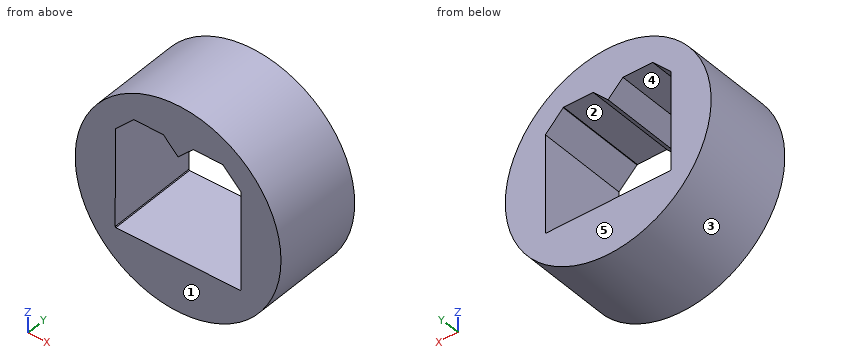
Autodesk Fusion 360 part; units mm, degrees
sketch "Sketch1" plane through (0, 0, 0) normal (0, 1, 0) x (1, 0, 0)
  circle A0 centre (0, 0) radius 6.5
  line L0 (10.0631, -5.0894) -> (15.2631, -5.0894)
  line L1 (15.2631, -5.0894) -> (15.2631, 5.1106)
  line L2 (15.2631, 5.1106) -> (10.0631, 5.1106)
  line L3 (10.0631, 5.1106) -> (10.0631, -5.0894)
  dimension "d1" = 13
  dimension "d2" = 5.2
  dimension "d3" = 10.2
sketch "Sketch2" plane through (0, 0, 0) normal (0, 1, 0) x (1, 0, 0)
sketch "Sketch3" plane through (0, 0, 0) normal (0, 1, 0) x (1, 0, 0)
  line L0 (-5.268, 4.2895) -> (-0.068, 4.2895)
  line L1 (-0.068, 4.2895) -> (-0.068, -3.9105)
  line L2 (-0.068, -3.9105) -> (-1.4822, -5.3247)
  line L3 (-0.068, -3.9105) -> (1.932, -3.9105) construction
  line L4 (-1.4822, -5.3247) -> (-3.8322, -5.3247)
  line L5 (-3.8322, -5.3247) -> (-5.2464, -3.9105)
  line L6 (-3.8322, -5.3247) -> (-1.9822, -5.3247) construction
  line L7 (-5.2464, -3.9105) -> (-5.268, 4.2895)
  line L8 (1.3678, -5.3247) -> (-0.0464, -3.9105)
  line L9 (5.132, 4.2895) -> (5.132, -3.9105)
  line L10 (-0.0464, -3.9105) -> (-0.068, 4.2895)
  line L11 (-0.068, 4.2895) -> (5.132, 4.2895)
  line L12 (5.132, -3.9105) -> (3.7178, -5.3247)
  line L13 (3.7178, -5.3247) -> (1.3678, -5.3247)
  line L14 (1.3678, -5.3247) -> (3.2178, -5.3247) construction
  line L15 (-5.2464, -3.9105) -> (5.132, 4.2895)
  line L16 (-5.268, 4.2895) -> (5.132, -3.9105)
  circle A0 centre (-0.068, 0.1895) radius 7
  line L17 (-5.268, 4.2895) -> (5.132, 4.2895)
  line L18 (-0.0464, -3.9105) -> (-0.068, -3.9105)
  circle A1 centre (-0.068, 0.1895) radius 9
  line L19 (-0.0572, -4.324) -> (-1.358, -5.6247)
  line L20 (-1.358, -5.6247) -> (-3.9565, -5.6247)
  line L21 (-3.9565, -5.6247) -> (-5.5461, -4.0351)
  line L22 (-5.5461, -4.0351) -> (-5.5688, 4.5895)
  line L23 (-5.5688, 4.5895) -> (-0.068, 4.5895)
  line L24 (-0.068, 4.5895) -> (5.432, 4.5895)
  line L25 (5.432, 4.5895) -> (5.432, -4.0348)
  line L26 (5.432, -4.0348) -> (3.842, -5.6247)
  line L27 (3.842, -5.6247) -> (1.2435, -5.6247)
  line L28 (1.2435, -5.6247) -> (-0.0572, -4.324)
  dimension "d4" = 5.2
  dimension "d5" = 8.2
  dimension "d6" = 135
  dimension "d7" = 2
  dimension "d8" = 2.35
  dimension "d9" = 135
  dimension "d10" = 2
  dimension "d11" = 5.2
  dimension "d12" = 8.2
  dimension "d13" = 2
  dimension "d14" = 2.35
  dimension "d15" = 135
  dimension "d16" = 2
  dimension "d17" = 14
  dimension "d20" = 18
  dimension "d27" = -0.3
extrude "Extrude2" add sketch "Sketch3" along normal blind 8 contours A0 L25 L26 | A0 L24 L25 | A0 L26 L27 | A0 L23 L24 | A0 L19 L20 L21 L22 L27 L28 | A0 L22 L23 | A1
Work out the finished part from the listing and answer in its coordinate system (mm). Face numbers are marked on the shaded views. A direction names the side the tool comes from. Give positions to 0.01 mm unless a question says otherwise; leave off trailing zeros. Order: outer loops, then holes, each group sorted by start corner. A loop starts at its lowest first (then second) coordinate and runs counter-clockwise, first axis right, second up.
1. Section B-B, the plane x = 0.25 is taken. Determine the outline of the cut face in (y, z).
Result sheet:
outline: (0, -9.18) - (8, -9.18) - (8, -4.59) - (0, -4.59) - close; (0, 4.63) - (8, 4.63) - (8, 8.8) - (0, 8.8) - close
2. Straight lines are drawn through the part: L1, parallel to Z at x = -3, y = 3.25; L2, parallel to X at y = 7.75, z = -4; L3, parallel to Z at x = -4, y = 6.5. For each, find the intervals that lie inside material, in ascending order.
Result sheet:
L1: z = -8.7 to -4.59, 5.62 to 8.32
L2: x = -8.22 to -5.57, 5.43 to 8.09
L3: z = -8.29 to -4.59, 5.58 to 7.91
3. The mould has two halves that part along X. Classify the marked faces 3, 4 and 5: released by +X, released by -X, zero draft, split by the parting line, or undercut.
Result sheet:
face 3: split by the parting line
face 4: undercut
face 5: zero draft
4. Each of these flat-tipped pins is pushed along its axis until it touches: P1, Ø1, axis at x = -4.5, y = 3, coming from the +Z side; P2, Ø1.3, axis at x = -3, y = 4, coming from the -Z side. Where does it stop, or does it pass through?
Result sheet:
P1: stops at z = 7.91
P2: stops at z = -8.9
5. Section D-D, the plane z = -7.75 is taken. Determine the outline of the cut face in (x, y).
Result sheet:
outline: (-4.95, 0) - (4.81, 0) - (4.81, 8) - (-4.95, 8) - close
6. Section A-A, the plane z = 3.25 is taken. Determine the outline of the cut face in (x, y), and give its area (3 significant figures).
Result sheet:
outline: (-8.38, 0) - (-5.55, 0) - (-5.55, 8) - (-8.38, 8) - close; (5.43, 0) - (8.25, 0) - (8.25, 8) - (5.43, 8) - close
area: 45.2 mm2
7. For the marked faces 1 and 2, determine the directions among +Z, -Z, +X, -X, +Y, -Y from which every point of the face is accessible in a straight line to the end or side of a thin tool.
Result sheet:
face 1: +Z, -Z, +X, -X, -Y
face 2: +Y, -Y
8. Section C-C, the plane y = 2.5 is taken. Determine the outline of the cut face in (x, z), and give its area (3 significant figures).
Result sheet:
outline: circle Ø18 at (-0.07, -0.19); hole (-5.57, -4.52) arc R7 ccw to (-5.51, -4.59) - (5.38, -4.59) arc R7 ccw to (5.43, -4.52) - (5.43, 4.03) - (3.87, 5.6) arc R7 ccw to (3.83, 5.62) - (1.24, 5.62) - (-0.06, 4.32) - (-1.36, 5.62) - (-3.96, 5.62) - (-5.55, 4.04) - close
area: 146 mm2
